Work out the finished part from the listing and answer in its coordinate system (mm). Face numbers are marked on the shaded views. A direction names the side the tool comes from. Round coordinates to 2 decimals unless told otherwise and drop trailing zeros. Write each loop counter-clockwise with the first axis right and the second up, starting at its lowest first coordinate (ties: lowest second). Pieces come first, ordered by that corner, then holes.
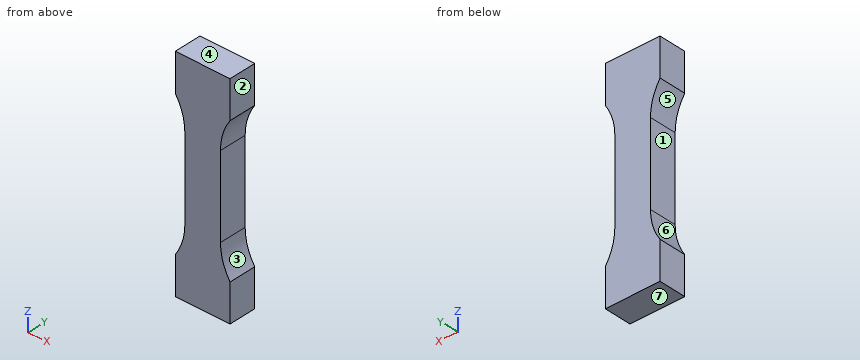
Autodesk Inventor part; units mm, degrees
ref_plane "YZ Plane" through (0, 0, 0) normal (1, 0, 0) x (0, 1, 0)
ref_plane "XZ Plane" through (0, 0, 0) normal (0, 1, 0) x (-1, 0, 0)
ref_plane "XY Plane" through (0, 0, 0) normal (0, 0, 1) x (1, 0, 0)
sketch "Sketch1" plane through (0, 0, 0) normal (0, 1, 0) x (-1, 0, 0)
  line L0 (0, 0) -> (20, 0)
  line L1 (3.5, 25) -> (3.5, 40)
  line L2 (16.5, 25) -> (16.5, 40)
  arc A0 (16.5, 25) -> (20, 13.6973) centre (36.5, 25) ccw
  arc A1 (0, 13.6973) -> (3.5, 25) centre (-16.5, 25) ccw
  line L3 (3.5, 40) -> (16.5, 40) construction
  line L4 (0, 13.6973) -> (0, 0)
  line L5 (20, 13.6973) -> (20, 0)
  line L6 (0, 80) -> (20, 80)
  line L7 (3.5, 55) -> (3.5, 40)
  line L8 (16.5, 55) -> (16.5, 40)
  arc A2 (20, 66.3027) -> (16.5, 55) centre (36.5, 55) ccw
  arc A3 (3.5, 55) -> (0, 66.3027) centre (-16.5, 55) ccw
  line L9 (0, 66.3027) -> (0, 80)
  line L10 (20, 66.3027) -> (20, 80)
  dimension "d2" = 20
  dimension "d5" = 20
  dimension "d6" = 20
  dimension "d7" = 40
  dimension "d8" = 13
  dimension "d9" = 15
  dimension "d13" = 15
extrude "Extrusion1" add sketch "Sketch1" along normal blind 10
properties part number "Generic DogBone"
Q1. Find section B-B (z = 37.5). Determine the outline of the cut face in (x, y), plus the area to 3 significant figures.
Q2. Find section A-A (y = 7). Determine the outline of the cut face in (x, z), plus the area to 3 significant figures.
Q3. A tool of negligible diameter and unlimited length cuts with its end or side. For the marked faces 1, 2 and 3, from which of +Z, -Z, +X, -X, +Y, -Y can it reach the whole face along a straight path? Write none if from no direction.
Q4. The mould has two halves that part along Z. Classify the marked faces 4, 5, 6 and 7: +Z half, -Z half, draft (parallel to the pull), parting line (faces both ways), or undercut.
Q5. Given pin 1 (5 mm diameter, centred on y = 6.5, z = 35.5, fed in from -X); pin 2 (3 mm diameter, centred on y = 3, z = 46, fed in from +X), each flat-ended and moving along its own axis, determine where each tip first touches the part or whether it passes through.
Q6. Find the intervals of material crossed by L1, parallel to X at y = 4.25, z = 34; L2, parallel to Z at x = -1.75, y = 6.75; L3, parallel to X at y = 3, z = 62 (3 decimals), in increasing order.
Q7. Find section C-C (z = 24). Determine the outline of the cut face in (x, y) (3 decimals), plus the area to 4 significant figures.
Report:
1. outline: (-16.5, 0) - (-3.5, 0) - (-3.5, 10) - (-16.5, 10) - close
1. area: 130 mm2
2. outline: (-20, 0) - (0, 0) - (0, 13.7) arc R20 cw to (-3.5, 25) - (-3.5, 55) arc R20 cw to (0, 66.3) - (0, 80) - (-20, 80) - (-20, 66.3) arc R20 cw to (-16.5, 55) - (-16.5, 25) arc R20 cw to (-20, 13.7) - close
2. area: 1,280 mm2
3. face 1: -X, +Y, -Y
3. face 2: +Z, -Z, +X, +Y, -Y
3. face 3: +X, +Y, -Y
4. face 4: +Z half
4. face 5: undercut
4. face 6: undercut
4. face 7: -Z half
5. pin 1: stops at x = -16.5
5. pin 2: stops at x = -3.5
6. L1: x = -16.5 to -3.5
6. L2: z = 0 to 16.82, 63.18 to 80
6. L3: x = -17.765 to -2.235
7. outline: (-16.525, 0) - (-3.475, 0) - (-3.475, 10) - (-16.525, 10) - close
7. area: 130.5 mm2
